Drawing for the job (mm, zero at the part's lowest x, y, z). Round coordinates to 2 decimals unless told otherwise and drop trailing zeros. Write each loop counter-clockwise with the first axis right and the second up, starting at its lowest first coordinate (ties: lowest second). Pieces come first, ordered by that corner, then holes.
Item 1: Mould opens along X. For the marked faces 1, 2 and 3 say: +X half, -X half, draft (parallel to the pull), parting line (faces both ways), or undercut.
Item 2: Band-saw the part on C-C, the plane z = 43.5. Write the cut outline in (x, y) (1 decimal).
Item 3: Wall check: probe 1 along Y at (x, z) = (38.1, 92) (1 decimal); probe 2 along X at (y, z) = (63, 64); probe 3 along Y at (x, z) = (36.5, 138). Give the ranges that are in metal, low to high.
Item 4: Band-saw the part on D-D, the plane y = 13. Write the cut outline in (x, z), then the cut area to 3 significant figures.
Item 5: Drop flat-ended pins along their axis: pin 1 Ø24 at (x, y) = (32.5, 62) entering from +Z; pin 2 Ø8 at (x, y) = (255, 94) entering from -Z; pin 3 Ø1 at (y, z) = (53.5, 91) entering from +X; pin 4 Ø10 at (x, z) = (62.5, 142.5) entering from -Y (1 decimal). Give the stop position or say it passes through.
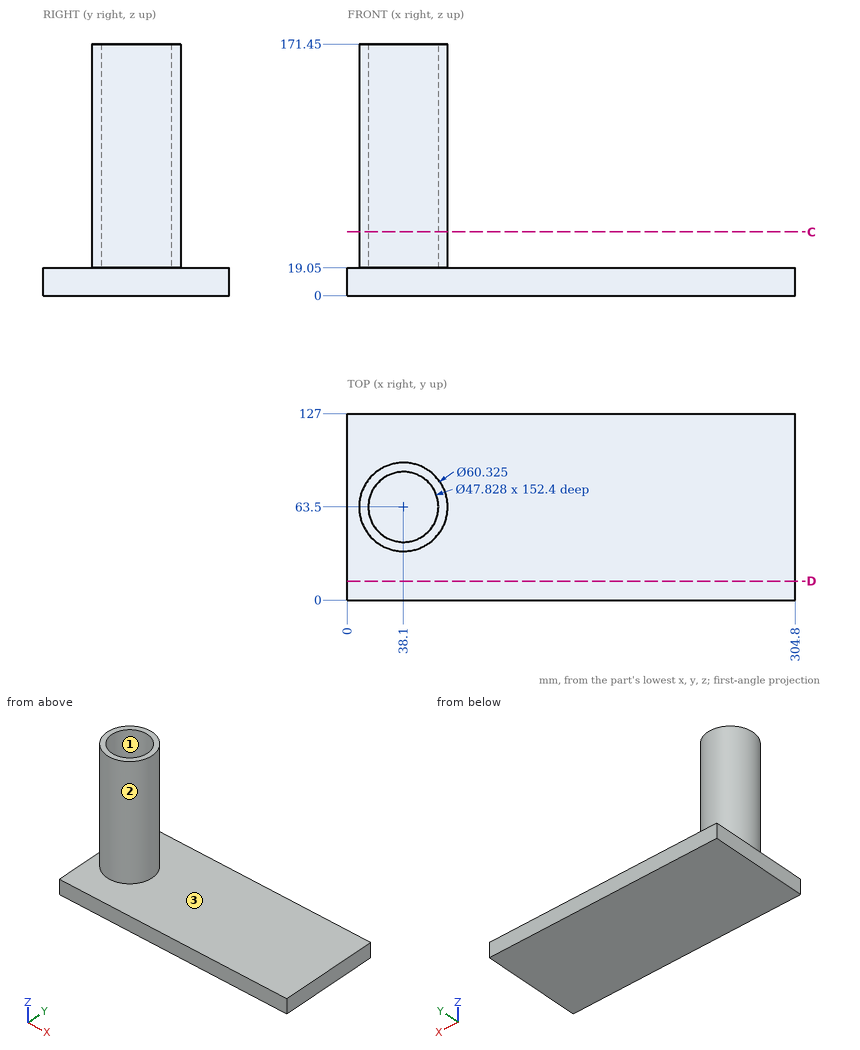
Results:
1. face 1: undercut
1. face 2: parting line
1. face 3: draft
2. outline: circle Ø60.3 at (38.1, 63.5); hole circle Ø47.8 at (38.1, 63.5)
3. probe 1: y = 33.3 to 39.6, 87.4 to 93.7
3. probe 2: x = 7.94 to 14.19, 62.01 to 68.26
3. probe 3: y = 33.38 to 39.64, 87.36 to 93.62
4. outline: (0, 0) - (304.8, 0) - (304.8, 19.05) - (0, 19.05) - close
4. area: 5,810 mm2
5. pin 1: stops at z = 19.05
5. pin 2: stops at z = 0
5. pin 3: stops at x = 66.73
5. pin 4: stops at y = 40.4
